from build123d import *

# Parameters (mm, degrees)
EXTRUDE_1_DEPTH     = 22
SKETCH_2_R          = 6
CUT_EXTRUDE_1_DEPTH = 112.39569112
SKETCH_3_R          = 3
CUT_EXTRUDE_2_DEPTH = 109.323589305


with BuildPart() as part:
    # ｽｹｯﾁ1 → ﾎﾞｽ - 押し出し1 (new body)
    with BuildSketch(Plane.XY):
        Polygon((-105, 15), (-105, 7), (-5, 7), (-5, -7), (-105, -7), (-105, -15), (0, -15), (0, 15), align=None)
    extrude(amount=EXTRUDE_1_DEPTH)

    # ｽｹｯﾁ2 → ｶｯﾄ - 押し出し1 (cut, through all)
    with BuildSketch(Plane.XZ.offset(15)):
        with Locations(Location((-94, 11, 0), (0, 0, 270))):
            Circle(SKETCH_2_R)
    extrude(amount=-CUT_EXTRUDE_1_DEPTH, mode=Mode.SUBTRACT)

    # ｽｹｯﾁ3 → ｶｯﾄ - 押し出し2 (cut, through all)
    with BuildSketch(Plane(origin=(0, 0, 0), x_dir=(0, 0, -1), z_dir=(1, 0, 0))):
        with Locations(Location((-11, 0, 0), (0, 0, 90))):
            Circle(SKETCH_3_R)
    extrude(amount=-CUT_EXTRUDE_2_DEPTH, mode=Mode.SUBTRACT)


solid = part.part
Geometry: final body of the model. Coordinates: model frame, mm. A direction names the side the tool comes from. Round coordinates to 2 decimals unless told otherwise and drop trailing zeros. Loops run counter-clockwise (first coordinate to the right, second up) from the corner with the lowest first, then second, coordinate; pieces in that order, holes last. Notation, with made-up numbers: M 0,48.25 L 43,48.25 A28 cw 43,84.25 Z; hole C 40.5,-37.5 d10. An arc over 180 degrees is marked long. One line per question, with ' | ' between items.
(1) Pull-direction query (Y, two-part tool) for faces 3 (the cylindrical face through (-2.465, 1.384, 8.338)), 4 (the flat face through (-52, 15, 11)), 5 (the flat face through (-53, 10, 22)); classes: +Y half, -Y half, draft (parallel to the pull), parting line (faces both ways), or undercut.
Check result:
face 3: undercut | face 4: +Y half | face 5: draft
(2) Cut plane D-D on z = 11. Return the cut outline in (x, y).
Check result:
outline: M -105,-15 L -100,-15 L -100,-7 L -105,-7 Z; M -105,7 L -100,7 L -100,15 L -105,15 Z; M -88,-15 L 0,-15 L 0,-3 L -5,-3 L -5,-7 L -88,-7 Z; M -88,7 L -5,7 L -5,3 L 0,3 L 0,15 L -88,15 Z
(3) Access query for faces 1 (the flat face through (-56, 7, 11)), 2 (the cylindrical face through (-88.941, 10.944, 7.774)). Directions: +Z, -Z, +X, -X, +Y, -Y. A direction counts if a zero-diameter tool reaches every point of the face in a straight line with its end or side. Return the directions, or none.
Check result:
face 1: +Z, -Z, -X | face 2: +Y, -Y
(4) Cut plane B-B on x = -83.5. Return the cut outline in (y, z), plus the area to 3 significant figures.
Check result:
outline: M -15,0 L -7,0 L -7,22 L -15,22 Z; M 7,0 L 15,0 L 15,22 L 7,22 Z | area: 352 mm2
(5) Material intervals for line 1 along Y through (x, z) = (-45, 19.25); line 2 along X through (y, z) = (-11.5, 11); line 3 along X through (y, z) = (-3.75, 9), sorted ascending. Write a range as from..to.
Check result:
line 1: y = -15..-7, 7..15 | line 2: x = -105..-100, -88..0 | line 3: x = -5..0
(6) Cut plane A-A on y = 0. Return the cut outline in (x, z), plus the area to 3 significant figures.
Check result:
outline: M -5,0 L 0,0 L 0,8 L -5,8 Z; M -5,14 L 0,14 L 0,22 L -5,22 Z | area: 80.0 mm2
(7) Cut plane C-C on x = -94. Return the cut outline in (y, z).
Check result:
outline: M -15,0 L -7,0 L -7,5 L -15,5 Z; M -15,17 L -7,17 L -7,22 L -15,22 Z; M 7,0 L 15,0 L 15,5 L 7,5 Z; M 7,17 L 15,17 L 15,22 L 7,22 Z
(8) Contact query for a flat-ended pin moving along its axis: P1, Ø3, axis at y = 5.5, z = 18, coming from the +X side. Output: stop coordinate, or through.
Check result:
P1: stops at x = 0
